Geometry check sheet. Reference: drawing and pictorial views, mm from the part's lowest x, y, z. Round coordinates to 2 decimals unless told otherwise and drop trailing zeros. Loops run counter-clockwise (first coordinate to the right, second up) from the corner with the lowest first, then second, coordinate; pieces in that order, holes last. Notation, with made-up numbers: (-11, -12.75) -> (48, -12.75) arc R32 ccw to (48, 13.25) -> close; hole circle Ø3 at (62, 78.25). An arc over 180 degrees is marked (long way). Use one line per item in the form item = value. Start each with the question number.
(1) Sectioned sample at D-D (y = 5.25). Record the cut outline in (x, z), and give its area (3 significant figures).
(2) Draft check along X on the marked faces 1, 2, 3 and 4. Enter one of: released by +X, released by -X, zero draft, split by the parting line, or undercut.
(3) Sectioned sample at C-C (x = 1.2). Record the cut outline in (y, z), and give its area (3 significant figures).
(4) Sectioned sample at B-B (y = 1.25). Record the cut outline in (x, z).
(5) Sectioned sample at A-A (z = 2.25). Record the cut outline in (x, y), and give its area (3 significant figures).
(6) Material ranges on probe 1 along Y at (x, z) = (1.2, 14.75); probe 2 along X at (y, z) = (1, 8); probe 3 along Z at (x, y) = (1.25, 5.25), recorded low to high. Write a range as [from, to].
(7) Go/stop test with flat-tipped pins: pin 1 (0.7 mm diameter, centred on y = 3.5, z = 1, fed in from +X); pin 2 (1 mm diameter, centred on x = 2, z = 10, fed in from -Y); pin 3 (1.5 mm diameter, centred on x = 1, y = 5, fed in from -Z). Record where each tip stops, or that it passes through.
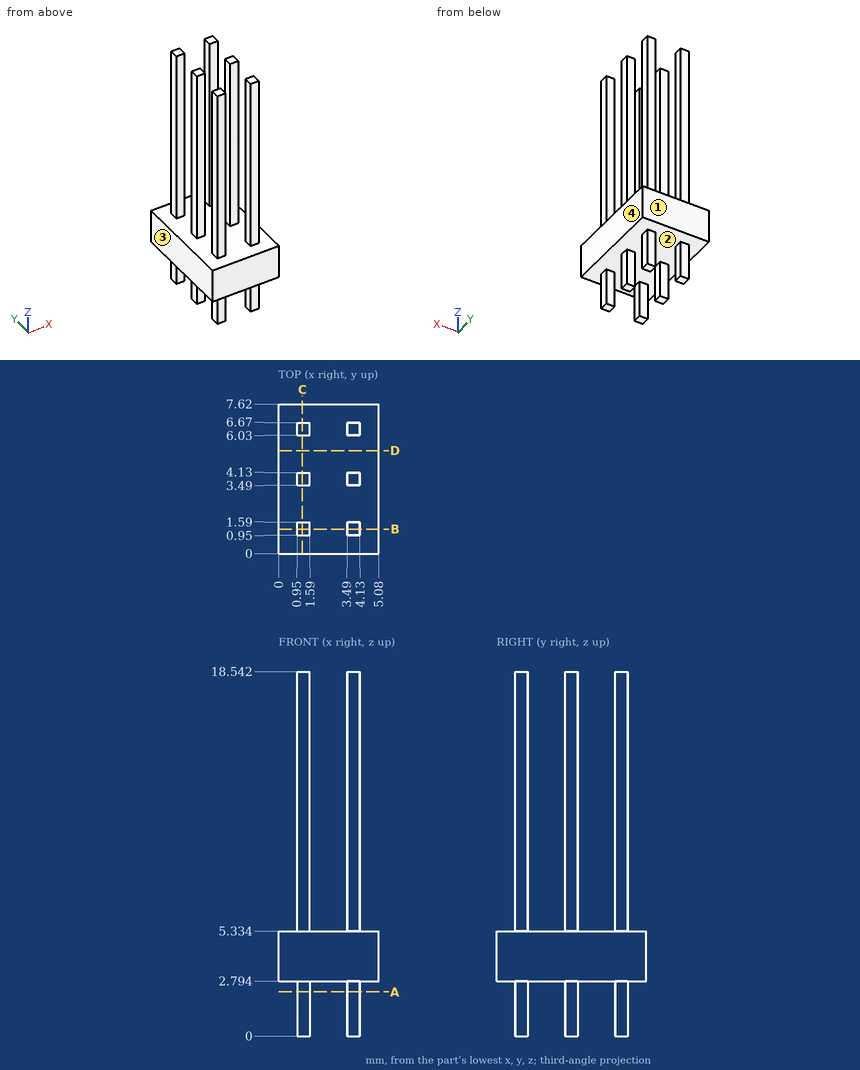
Checks:
q1.outline = (0, 2.79) -> (5.08, 2.79) -> (5.08, 5.33) -> (0, 5.33) -> close
q1.area = 12.9 mm2
q2.face_1 = zero draft
q2.face_2 = undercut
q2.face_3 = released by -X
q2.face_4 = released by +X
q3.outline = (0, 2.79) -> (0.95, 2.79) -> (0.95, 0) -> (1.59, 0) -> (1.59, 2.79) -> (3.49, 2.79) -> (3.49, 0) -> (4.13, 0) -> (4.13, 2.79) -> (6.03, 2.79) -> (6.03, 0) -> (6.67, 0) -> (6.67, 2.79) -> (7.62, 2.79) -> (7.62, 5.33) -> (6.67, 5.33) -> (6.67, 18.54) -> (6.03, 18.54) -> (6.03, 5.33) -> (4.13, 5.33) -> (4.13, 18.54) -> (3.49, 18.54) -> (3.49, 5.33) -> (1.59, 5.33) -> (1.59, 18.54) -> (0.95, 18.54) -> (0.95, 5.33) -> (0, 5.33) -> close
q3.area = 50.1 mm2
q4.outline = (0, 2.79) -> (0.95, 2.79) -> (0.95, 0) -> (1.59, 0) -> (1.59, 2.79) -> (3.49, 2.79) -> (3.49, 0) -> (4.13, 0) -> (4.13, 2.79) -> (5.08, 2.79) -> (5.08, 5.33) -> (4.13, 5.33) -> (4.13, 18.54) -> (3.49, 18.54) -> (3.49, 5.33) -> (1.59, 5.33) -> (1.59, 18.54) -> (0.95, 18.54) -> (0.95, 5.33) -> (0, 5.33) -> close
q5.outline = (0.95, 0.95) -> (1.59, 0.95) -> (1.59, 1.59) -> (0.95, 1.59) -> close; (0.95, 3.49) -> (1.59, 3.49) -> (1.59, 4.13) -> (0.95, 4.13) -> close; (0.95, 6.03) -> (1.59, 6.03) -> (1.59, 6.67) -> (0.95, 6.67) -> close; (3.49, 0.95) -> (4.13, 0.95) -> (4.13, 1.59) -> (3.49, 1.59) -> close; (3.49, 3.49) -> (4.13, 3.49) -> (4.13, 4.13) -> (3.49, 4.13) -> close; (3.49, 6.03) -> (4.13, 6.03) -> (4.13, 6.67) -> (3.49, 6.67) -> close
q5.area = 2.46 mm2
q6.probe_1 = [0.95, 1.59], [3.49, 4.13], [6.03, 6.67]
q6.probe_2 = [0.95, 1.59], [3.49, 4.13]
q6.probe_3 = [2.79, 5.33]
q7.pin_1 = 4.13
q7.pin_2 = 0.95
q7.pin_3 = 2.79
